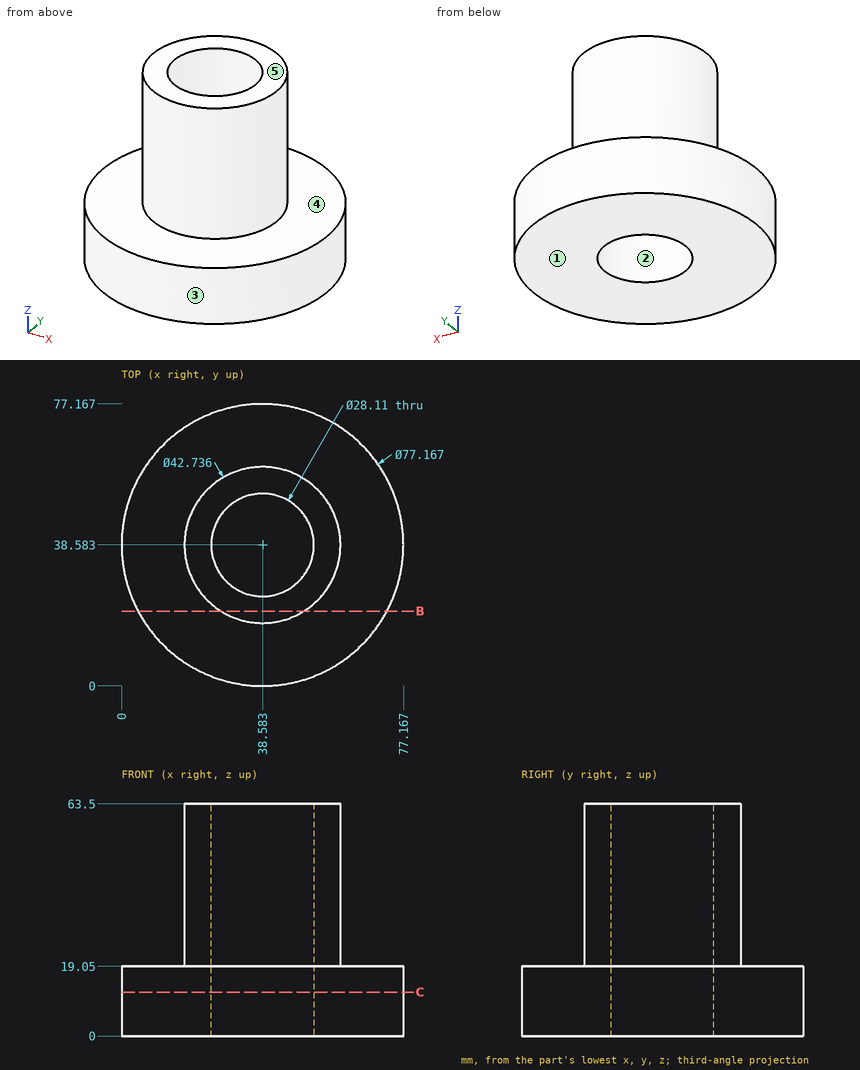
Job drawing, mm, ordinate dimensions from the low corner. One solid piece. A direction names the side the tool comes from. Coordinates: 2 decimals unless noted, no trailing zeros. Loops run counter-clockwise (first coordinate to the right, second up) from the corner with the lowest first, then second, coordinate; pieces in that order, holes last. Notation, with made-up numbers: (-18.5, -16) - (-14.5, -16) arc R27 cw to (-14.5, 21) - close; hole circle Ø11 at (20.25, 78). An arc over 180 degrees is marked (long way). Write item = value, one per line. Start each with the question number.
Q1. Drill centre lines: L1, parallel to Z at x = 55, y = 61; L2, parallel to X at y = 39, z = 53 (1 decimal); L3, parallel to Y at x = 49.5, z = 12 (1 decimal). Where is each one in solid material? Low to high.
Q2. Pull direction Y, two halves, no side cores. Call the marked faces 1, 2 and 3: pulls with the +Y half, pulls with the -Y half, needs draft (parallel to the pull), parting line crosses it, or undercut.
Q3. Cut at C-C, the plane z = 12. List the corners of the cut face in (x, y) (1 decimal), then the cut area to 3 significant figures.
Q4. Flat gauge pins, fed straight in: pin 1 Ø12 at (x, z) = (55.5, 9) entering from +Y; pin 2 Ø12 at (x, z) = (34, 37.5) entering from +Y; pin 3 Ø3 at (x, z) = (57, 49) entering from -Y. Where does each tip first touch, or does it go through?
Q5. Which spindle directions (+Z, -Z, +X, -X, +Y, -Y) get a long thin tool onto all of the face, cutting with end or side? Do the marked faces 4 and 5. Say none if no direction does.
Q6. Cut at B-B, the plane y = 20.5. List the corners of the cut face in (x, z).
Computed:
q1.L1 = 0 to 19.05
q1.L2 = 17.2 to 24.5, 52.6 to 59.9
q1.L3 = 1.6 to 29.7, 47.4 to 75.6
q2.face_1 = needs draft
q2.face_2 = undercut
q2.face_3 = parting line crosses it
q3.outline = circle Ø77.2 at (38.6, 38.6); hole circle Ø28.1 at (38.6, 38.6)
q3.area = 4,060 mm²
q4.pin_1 = 75.59
q4.pin_2 = 59.95
q4.pin_3 = 25.53
q5.face_4 = +Z
q5.face_5 = +Z, +X, -X, +Y, -Y
q6.outline = (4.5, 0) - (72.67, 0) - (72.67, 19.05) - (49.97, 19.05) - (49.97, 63.5) - (27.2, 63.5) - (27.2, 19.05) - (4.5, 19.05) - close
